from build123d import *

# Parameters (mm, degrees)
SKETCH1_W              = 80
SKETCH1_H              = 28.75
BOSS_EXTRUDE1_DEPTH    = 6
M5_CLEARANCE_HOLE1_D   = 5.5
M1_6_CLEARANCE_HOLE1_D = 1.7
CUT_EXTRUDE1_START     = -6
SKETCH9_W              = 29.5
SKETCH9_H              = 23.753520778
CUT_EXTRUDE1_DEPTH     = 2
FILLET1_R              = 2
FILLET2_R              = 3


with BuildPart() as part:
    # Sketch1 → Boss-Extrude1 (new body)
    with BuildSketch(Plane(origin=(0, 0, 0), x_dir=(0, 0, -1), z_dir=(1, 0, 0))):
        Rectangle(SKETCH1_W, SKETCH1_H)
    extrude(amount=BOSS_EXTRUDE1_DEPTH)

    # M5 Clearance Hole1 (through all)
    with Locations(Plane.ZY):
        with Locations((-33.5, 3.125), (23.5, 3.125)):
            Hole(M5_CLEARANCE_HOLE1_D / 2)

    # M1.6 Clearance Hole1 (through all)
    with Locations(Plane.ZY):
        with Locations((-10.25, -0.975), (10.25, -0.975), (0, -0.975), (-5.125, -9.851760389), (5.125, -9.851760389), (5.125, 7.901760389), (-5.125, 7.901760389)):
            Hole(M1_6_CLEARANCE_HOLE1_D / 2)

    # Sketch9 → Cut-Extrude1 (cut)
    with BuildSketch(Plane(origin=(6, 0, 0), x_dir=(0, 0, -1), z_dir=(1, 0, 0)).offset(CUT_EXTRUDE1_START)):
        with Locations((0, -0.975)):
            Rectangle(SKETCH9_W, SKETCH9_H)
    extrude(amount=CUT_EXTRUDE1_DEPTH, mode=Mode.SUBTRACT)

    # Fillet1
    fillet1_edges = [part.edges().sort_by_distance(p)[0] for p in [
        (1, -12.851760389, 14.75),
        (1, -12.851760389, -14.75),
        (1, 10.901760389, -14.75),
        (1, 10.901760389, 14.75),
    ]]
    fillet(fillet1_edges, radius=FILLET1_R)

    # Fillet2
    fillet2_edges = [part.edges().sort_by_distance(p)[0] for p in [
        (3, -14.375, -40),
        (3, -14.375, 40),
        (3, 14.375, 40),
        (3, 14.375, -40),
    ]]
    fillet(fillet2_edges, radius=FILLET2_R)


solid = part.part
Design review of the part built by this model. Coordinates are the model's own, in mm. A direction names the side the tool comes from. Give positions to 0.01 mm unless a question says otherwise; leave off trailing zeros. Loops run counter-clockwise (first coordinate to the right, second up) from the corner with the lowest first, then second, coordinate; pieces in that order, holes last. Notation, with made-up numbers: (66.25, 14) -> (72.25, 14) arc R16 cw to (72.25, 25) -> close; hole circle Ø8 at (-4, 83). An arc over 180 degrees is marked (long way). One line per question, with ' | ' between items. Start each with the question number.
(1) Draft analysis for pull direction Y (two halves, no side actions). For faces 3 (the face through (1, -12.852, 0)), 4 (the face through (3.042, 13.473, 39.145)), 5 (the face through (3.04, -13.52, -39.1)), state which applies: +Y half, -Y half, draft (parallel to the pull), parting line (faces both ways), or undercut.
(2) For faces 1 (the face through (3.042, -13.473, 39.145)), 2 (the face through (1, -1, 14.75)), list the 3-axis set-ups (+Z, -Z, +X, -X, +Y, -Y) from which the entire face can be reached by the end or side of a thin tool; tool diameter is ignored.
(3) We need section A-A (z = 0). State the section outline as (x, y) points (3 decimals).
(4) Insertion check: P1, Ø1, axis at y = 7.9, z = -5.12, coming from the -X side; P2, Ø2.5, axis at y = -0.975, z = 0, coming from the -X side. Each pin has a flat end and moves straight along its axis. Give the tip position at first contact, or say it passes through.
(5) We need section B-B (x = 4.25). State how many separate pieces and enclosed holes the cut face has, and give its area (3 significant figures).
(6) We need section C-C (y = -3.75). State the section outline as (x, z) points, and give its area (3 significant figures).
(7) We need section D-D (y = 4.25). State the section outline as (x, z) points, and give its area (3 significant figures).
(8) For line 1 (Z direction, x = 3, y = 7.75); line 2 (Y direction, x = 5.5, z = -5) (3 decimals); line 3 (Y direction, x = 4.5, z = 10.25) (3 decimals), list the stretches that pass through material, from the lowest coordinate up.
The answers:
1) face 3: undercut | face 4: +Y half | face 5: -Y half
2) face 1: +Z, +X, -X, -Y | face 2: -X
3) outline: (0, -14.375) -> (6, -14.375) -> (6, -1.825) -> (2, -1.825) -> (2, -12.852) -> (0, -12.852) -> close; (0, 10.902) -> (2, 10.902) -> (2, -0.125) -> (6, -0.125) -> (6, 14.375) -> (0, 14.375) -> close
4) P1: passes through | P2: stops at x = 2
5) separate pieces: 1 | enclosed holes: 9 | area: 2,230 mm^2
6) outline: (0, -40) -> (6, -40) -> (6, 40) -> (0, 40) -> (0, 14.75) -> (2, 14.75) -> (2, -14.75) -> (0, -14.75) -> close | area: 421 mm^2
7) outline: (0, -40) -> (6, -40) -> (6, -36.01) -> (0, -36.01) -> close; (0, -30.99) -> (6, -30.99) -> (6, 20.99) -> (0, 20.99) -> (0, 14.75) -> (2, 14.75) -> (2, -14.75) -> (0, -14.75) -> close; (0, 26.01) -> (6, 26.01) -> (6, 40) -> (0, 40) -> close | area: 361 mm^2
8) line 1: z = -40 to -5.96, -4.29 to 4.29, 5.96 to 40 | line 2: y = -14.375 to -10.693, -9.011 to 7.061, 8.743 to 14.375 | line 3: y = -14.375 to -1.825, -0.125 to 14.375
